from build123d import *

# Parameters (mm, degrees)
SKETCH1_R           = 12.5
BOSS_EXTRUDE1_DEPTH = 38
SKETCH2_R           = 6
CUT_EXTRUDE1_DEPTH  = 76
CUT_EXTRUDE2_REACH  = 137.44
SKETCH3_R           = 12.5
CHAMFER1_SIZE       = 13


with BuildPart() as part:
    # Sketch1 → Boss-Extrude1 (new, symmetric)
    with BuildSketch(Plane(origin=(0, 0, 0), x_dir=(0, 0, -1), z_dir=(1, 0, 0))):
        with BuildLine():
            Line((0, 25), (-64, 25))
            Line((-64, 25), (-64, 9))
            Line((-64, 9), (-23.323807579, 9))
            ThreePointArc((-23.323807579, 9), (-20.615528128, -14.142135624), (0, -25))
            Line((0, -25), (56, -25))
            Line((56, -25), (56, 50))
            Line((56, 50), (40, 50))
            Line((40, 50), (40, -9))
            Line((40, -9), (23.323807579, -9))
            ThreePointArc((23.323807579, -9), (20.615528128, 14.142135624), (0, 25))
        make_face()
        Circle(SKETCH1_R, mode=Mode.SUBTRACT)
    extrude(amount=BOSS_EXTRUDE1_DEPTH, both=True)

    # Sketch2 → Cut-Extrude1 (cut)
    with BuildSketch(Plane(origin=(0, 25, 0), x_dir=(1, 0, 0), z_dir=(0, 1, 0))):
        with Locations(Location((-22, -48, 0), (0, 0, 270))):
            Circle(SKETCH2_R)
        with Locations(Location((22, -48, 0), (0, 0, 270))):
            Circle(SKETCH2_R)
    extrude(amount=-CUT_EXTRUDE1_DEPTH, mode=Mode.SUBTRACT)

    # Sketch3 → Cut-Extrude2 (cut, up to next)
    with BuildSketch(Plane(origin=(0, 0, -56), x_dir=(-1, 0, 0), z_dir=(0, 0, -1)), mode=Mode.PRIVATE) as cut_extrude2_sk1:
        with Locations((0, 18)):
            Circle(SKETCH3_R)
    cut_extrude2_tool1 = extrude(cut_extrude2_sk1.sketch, amount=-CUT_EXTRUDE2_REACH, mode=Mode.PRIVATE) & part.part
    add(cut_extrude2_tool1.solids().sort_by_distance((0, 18, -56))[0], mode=Mode.SUBTRACT)

    # Chamfer1
    chamfer1_edges = [part.edges().sort_by_distance(p)[0] for p in [
        (-38, 50, -48),
        (38, 50, -48),
    ]]
    chamfer(chamfer1_edges, length=CHAMFER1_SIZE)


solid = part.part
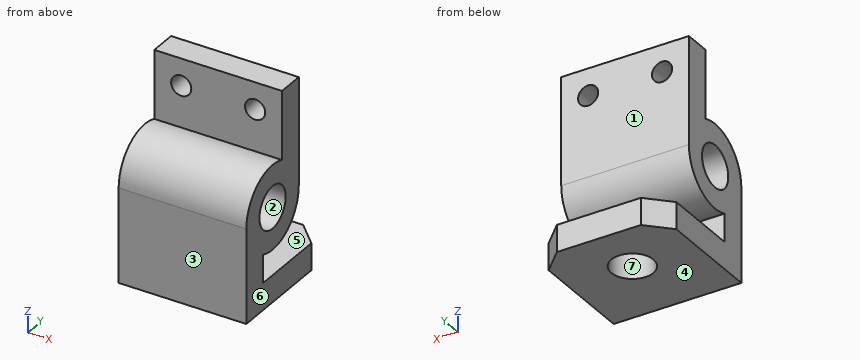
Geometry: final body of the model. Coordinates: model frame, mm. Face numbers are marked on the shaded views. A direction names the side the tool comes from. Coordinates: 2 decimals unless noted, no trailing zeros. Loops run counter-clockwise (first coordinate to the right, second up) from the corner with the lowest first, then second, coordinate; pieces in that order, holes last. Notation, with made-up numbers: (38.5, 79.25) - (47.5, 79.25) arc R20 cw to (47.5, 113.25) - close; hole circle Ø10 at (55.25, -39). An arc over 180 degrees is marked (long way). Put each result on its own line as item: value. Start each with the question number.
Q1. Cut plane B-B, the plane z = 48. Return loops of the section in (x, y).
Q2. Line query: line 1 (X direction, y = 20, z = 48); line 2 (Y direction, x = 0, z = -49); line 3 (Y direction, x = -14.5, z = 57). Output: solid intervals per line, ascending.
Q3. Cut plane A-A, the plane x = 0. Return loops of the section in (y, z).
Q4. Cut plane D-D, the plane z = -47.5. Return loops of the section in (x, y), and give its area (3 significant figures).
Q5. Pin query (flat end, axial travel): pin 1 Ø19 at (x, z) = (9.5, 28.5) entering from +Y; pin 2 Ø19 at (x, z) = (-22, 48) entering from -Y; pin 3 Ø6 at (x, z) = (10, -31.5) entering from +Y; pin 4 Ø11 at (x, z) = (22, 48) entering from +Y. Return the tip coordinate at first contact, or that it passes through.
Q6. Cut plane C-C, the plane y = 0. Return loops of the section in (x, z).
Q7. Set-up query: the marked faces 5, 6 and 7. Return all of +Z, -Z, +X, -X, +Y, -Y with unobstructed straight access to the full face (end or side cutting, diameter ignored); none if empty.
Q8. Pull-direction query (Y, two-part tool) for the marked faces 1, 2, 3 and 4; classes: released by +Y, released by -Y, zero draft, split by the parting line, or undercut.
Filled sheet:
1. outline: (-38, 9) - (-28, 9) - (-28, 25) - (-38, 25) - close; (-16, 9) - (16, 9) - (16, 25) - (-16, 25) - close; (28, 9) - (38, 9) - (38, 25) - (28, 25) - close
2. line 1: -38 to -28, -16 to 16, 28 to 38
2. line 2: -25 to 5.5, 30.5 to 50
2. line 3: 9 to 25
3. outline: (-25, -56) - (5.5, -56) - (5.5, -40) - (-9, -40) - (-9, -23.32) arc R25 ccw to (25, 0) - (25, 64) - (9, 64) - (9, 23.32) arc R25 ccw to (-25, 0) - close; (30.5, -56) - (50, -56) - (50, -40) - (30.5, -40) - close; hole circle Ø25 at (0, 0)
4. outline: (-38, -25) - (38, -25) - (38, 37) - (25, 50) - (-25, 50) - (-38, 37) - close; hole circle Ø25 at (0, 18)
4. area: 5,040 mm²
5. pin 1: y = 25
5. pin 2: y = 9
5. pin 3: y = -9
5. pin 4: through
6. outline: (-38, -56) - (38, -56) - (38, -40) - (-38, -40) - close; (-38, -25) - (38, -25) - (38, -12.5) - (-38, -12.5) - close; (-38, 12.5) - (38, 12.5) - (38, 25) - (-38, 25) - close
7. face 5: +X, -X, +Y
7. face 6: +Z, -Z, +X, +Y, -Y
7. face 7: -Z
8. face 1: released by +Y
8. face 2: undercut
8. face 3: released by -Y
8. face 4: zero draft
